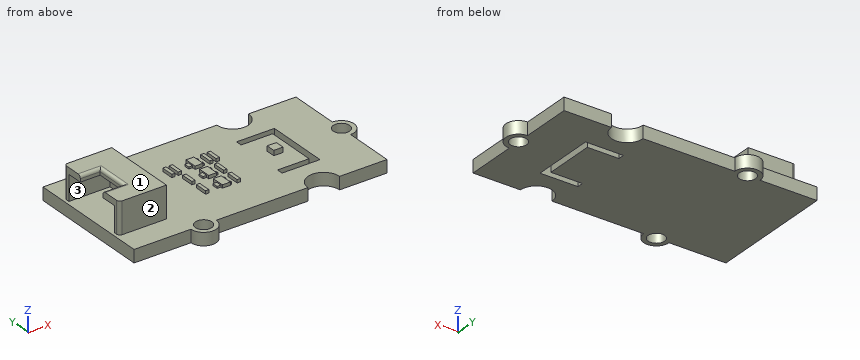
from build123d import *

# Parameters (mm, degrees)
SKETCH1_R           = 1.3
BOSS_EXTRUDE1_DEPTH = 2
BOSS_EXTRUDE2_DEPTH = 5
SKETCH3_W           = 4
SKETCH3_H           = 10
CUT_EXTRUDE1_DEPTH  = 7
SKETCH4_W           = 5
SKETCH4_H           = 12
CUT_EXTRUDE2_DEPTH  = 0.5
CUT_EXTRUDE3_DEPTH  = 1.5
FILLET1_R           = 0.5
SKETCH6_W           = 1.450763296
SKETCH6_H           = 1.450763296
BOSS_EXTRUDE3_DEPTH = 0.8
SKETCH7_W           = 0.528041157
SKETCH7_H           = 2.003611801
BOSS_EXTRUDE4_DEPTH = 0.5
SKETCH8_W           = 1.250632541
SKETCH8_H           = 2.003611801
BOSS_EXTRUDE5_DEPTH = 0.5
SKETCH9_W           = 0.587023474
SKETCH9_H           = 0.894026868
SKETCH9_W_2         = 0.333695167
SKETCH9_H_2         = 0.350698787
SKETCH9_W_3         = 0.333695166
SKETCH9_H_3         = 0.390012219
SKETCH9_H_4         = 0.39001222
SKETCH9_H_5         = 0.350698788
BOSS_EXTRUDE6_DEPTH = 0.3


with BuildPart() as part:
    # Sketch1 → Boss-Extrude1 (new body)
    with BuildSketch(Plane.XY):
        with BuildLine():
            Line((0, 0), (9, 0))
            ThreePointArc((9, 0), (11, -2), (13, 0))
            Line((13, 0), (27.5, 0))
            ThreePointArc((27.5, 0), (30, 2.5), (32.5, 0))
            Line((32.5, 0), (40, 0))
            Line((40, 0), (40, 8))
            ThreePointArc((40, 8), (42, 10), (40, 12))
            Line((40, 12), (40, 20))
            Line((40, 20), (32.5, 20))
            ThreePointArc((32.5, 20), (30, 17.5), (27.5, 20))
            Line((27.5, 20), (13, 20))
            ThreePointArc((13, 20), (11, 22), (9, 20))
            Line((9, 20), (0, 20))
            Line((0, 20), (0, 0))
        make_face()
        with Locations((11, 20)):
            Circle(SKETCH1_R, mode=Mode.SUBTRACT)
        with Locations((11, 0)):
            Circle(SKETCH1_R, mode=Mode.SUBTRACT)
        with Locations((40, 10)):
            Circle(SKETCH1_R, mode=Mode.SUBTRACT)
        Polygon((33, 15), (27, 15), (27, 14), (32, 14), (32, 6), (27, 6), (27, 5), (33, 5), align=None, mode=Mode.SUBTRACT)
    extrude(amount=BOSS_EXTRUDE1_DEPTH)

    # Sketch2 → Boss-Extrude2 (add)
    with BuildSketch(Plane.XY.offset(2)):
        Polygon((0, 10), (0, 16), (8, 16), (8, 4), (0, 4), align=None)
    extrude(amount=BOSS_EXTRUDE2_DEPTH)

    # Sketch3 → Cut-Extrude1 (cut)
    with BuildSketch(Plane.ZY):
        with Locations((4, 10)):
            Rectangle(SKETCH3_W, SKETCH3_H)
    extrude(amount=-CUT_EXTRUDE1_DEPTH, mode=Mode.SUBTRACT)

    # Sketch4 → Cut-Extrude2 (cut)
    with BuildSketch(Plane.ZY):
        with Locations((4.5, 10)):
            Rectangle(SKETCH4_W, SKETCH4_H)
    extrude(amount=-CUT_EXTRUDE2_DEPTH, mode=Mode.SUBTRACT)

    # Sketch5 → Cut-Extrude3 (cut)
    with BuildSketch(Plane.XY.offset(7)):
        Polygon((3.638822155, 12.5), (0.5, 12.5), (0.5, 10), (0.5, 7.5), (3.638822155, 7.5), align=None)
    extrude(amount=-CUT_EXTRUDE3_DEPTH, mode=Mode.SUBTRACT)

    # Fillet1
    fillet1_edges = [part.edges().sort_by_distance(p)[0] for p in [
        (0.5, 4, 4.5),
        (0.5, 16, 4.5),
        (2.069411077, 7.5, 7),
        (3.638822155, 10, 7),
        (2.069411077, 12.5, 7),
    ]]
    fillet(fillet1_edges, radius=FILLET1_R)

    # Sketch6 → Boss-Extrude3 (add)
    with BuildSketch(Plane.XY.offset(2)):
        with Locations((29.5, 10)):
            Rectangle(SKETCH6_W, SKETCH6_H)
    extrude(amount=BOSS_EXTRUDE3_DEPTH)

    # Sketch7 → Boss-Extrude4 (add)
    with BuildSketch(Plane.XY.offset(2)):
        with Locations((16.091644497, 13.2872497)):
            Rectangle(SKETCH7_W, SKETCH7_H)
        with Locations((15.091644497, 13.2872497)):
            Rectangle(SKETCH7_W, SKETCH7_H)
        with Locations((16.091644497, 10.2872497)):
            Rectangle(SKETCH7_W, SKETCH7_H)
        with Locations((16.091644497, 7.2872497)):
            Rectangle(SKETCH7_W, SKETCH7_H)
        with Locations((22.091644497, 13.2872497)):
            Rectangle(SKETCH7_W, SKETCH7_H)
        with Locations((21.091644497, 13.2872497)):
            Rectangle(SKETCH7_W, SKETCH7_H)
        with Locations((21.091644497, 10.2872497)):
            Rectangle(SKETCH7_W, SKETCH7_H)
        with Locations((21.091644497, 7.2872497)):
            Rectangle(SKETCH7_W, SKETCH7_H)
    extrude(amount=BOSS_EXTRUDE4_DEPTH)

    # Sketch8 → Boss-Extrude5 (add)
    with BuildSketch(Plane.XY.offset(2)):
        with Locations((19.1224917, 10.2872497)):
            Rectangle(SKETCH8_W, SKETCH8_H)
        with Locations((19.1224917, 13.2872497)):
            Rectangle(SKETCH8_W, SKETCH8_H)
        with Locations((19.1224917, 7.2872497)):
            Rectangle(SKETCH8_W, SKETCH8_H)
    extrude(amount=BOSS_EXTRUDE5_DEPTH)

    # Sketch9 → Boss-Extrude6 (add)
    with BuildSketch(Plane.XY.offset(2)):
        with Locations((18.203663692, 13.292407159)):
            Rectangle(SKETCH9_W, SKETCH9_H)
        with Locations((18.203663692, 10.192407159)):
            Rectangle(SKETCH9_W, SKETCH9_H)
        with Locations((18.203663692, 7.092407159)):
            Rectangle(SKETCH9_W, SKETCH9_H)
        with Locations((19.914655554, 13.914769987)):
            Rectangle(SKETCH9_W_2, SKETCH9_H_2)
        with Locations((19.921649724, 9.650395769)):
            Rectangle(SKETCH9_W_3, SKETCH9_H_3)
        with Locations((19.914655554, 12.650387615)):
            Rectangle(SKETCH9_W_2, SKETCH9_H_4)
        with Locations((19.921649724, 10.91477814)):
            Rectangle(SKETCH9_W_3, SKETCH9_H_5)
        with Locations((19.928643894, 6.650403922)):
            Rectangle(SKETCH9_W_3, SKETCH9_H_3)
        with Locations((19.928643894, 7.914786293)):
            Rectangle(SKETCH9_W_3, SKETCH9_H_5)
    extrude(amount=BOSS_EXTRUDE6_DEPTH)


solid = part.part
Read the model definition and answer for the solid it produces. Units are mm, in the model's axes. Face numbers are marked on the shaded views. Round coordinates to 2 decimals unless told otherwise and drop trailing zeros. Order: outer loops, then holes, each group sorted by start corner. A loop starts at its lowest first (then second) coordinate and runs counter-clockwise, first axis right, second up.
1) Straight lines are drawn through the part: L1, parallel to Y at x = 11, z = 1.2; L2, parallel to Z at x = 5, y = 13.75; L3, parallel to Z at x = 39, y = 19. For each, find the intervals that lie inside material, in ascending order.
2) The part is cut by section C-C on z = 1.25. Write down the section's boundary in (x, y).
3) The part is cut by section B-B on x = 5. Write down the section's boundary in (y, z).
4) Flat-ended cylindrical pins translate along their axes: pin 1 (3 mm diameter, centred on x = 3, z = 5, fed in from +Y); pin 2 (0.6 mm diameter, centred on x = 18.5, y = 13, fed in from +Z); pin 3 (0.6 mm diameter, centred on x = 29.5, z = 2.5, fed in from +Y); pin 4 (0.6 mm diameter, centred on y = 13.5, z = 2, fed in from -X). Find the tip coordinate at first contact, or state that the pin passes through.
5) The part is cut by section A-A on x = 11. Write down the section's boundary in (y, z), plus the area to 3 significant figures.
6) The mould has two halves that part along Y. Classify the marked faces 1, 2 and 3: released by +Y, released by -Y, zero draft, split by the parting line, or undercut.
7) The part is cut by section D-D on z = 5.25. Write down the section's boundary in (x, y).
Resolved:
1. L1: y = -2 to -1.3, 1.3 to 18.7, 21.3 to 22
1. L2: z = 0 to 2, 6 to 7
1. L3: z = 0 to 2
2. outline: (0, 0) - (9, 0) arc R2 ccw to (13, 0) - (27.5, 0) arc R2.5 cw to (32.5, 0) - (40, 0) - (40, 8) arc R2 ccw to (40, 12) - (40, 20) - (32.5, 20) arc R2.5 cw to (27.5, 20) - (13, 20) arc R2 ccw to (9, 20) - (0, 20) - close; hole circle Ø2.6 at (11, 0); hole circle Ø2.6 at (11, 20); hole (27, 5) - (33, 5) - (33, 15) - (27, 15) - (27, 14) - (32, 14) - (32, 6) - (27, 6) - close; hole circle Ø2.6 at (40, 10)
3. outline: (0, 0) - (20, 0) - (20, 2) - (16, 2) - (16, 7) - (4, 7) - (4, 2) - (0, 2) - close; hole (5, 2) - (15, 2) - (15, 6) - (5, 6) - close
4. pin 1: stops at y = 16
4. pin 2: stops at z = 2.5
4. pin 3: stops at y = 10.73
4. pin 4: stops at x = 0
5. outline: (-2, 0) - (-1.3, 0) - (-1.3, 2) - (-2, 2) - close; (1.3, 0) - (18.7, 0) - (18.7, 2) - (1.3, 2) - close; (21.3, 0) - (22, 0) - (22, 2) - (21.3, 2) - close
5. area: 37.6 mm2
6. face 1: zero draft
6. face 2: released by -Y
6. face 3: undercut
7. outline: (0.5, 4.5) arc R0.5 ccw to (1, 4) - (8, 4) - (8, 16) - (1, 16) arc R0.5 ccw to (0.5, 15.5) - (0.5, 15) - (7, 15) - (7, 5) - (0.5, 5) - close
